Could you check a few things on this drawing? It's one solid part, dimensions in mm from its lowest x, y, z. A direction names the side the tool comes from. Give positions to 0.01 mm unless a question says otherwise; leave off trailing zeros. Write each loop counter-clockwise with the first axis right and the second up, starting at its lowest first coordinate (ties: lowest second). Pieces come first, ordered by that corner, then holes. Notation, with made-up numbers: (-16, 54) -> (2, 54) arc R34 cw to (2, 85) -> close; hole circle Ø9 at (61, -33). An arc over 180 degrees is marked (long way). Use CSV: the item, a comma, the result in double quotes. Start each with the question number.
(1) For pin 1 Ø3.5 at (y, z) = (20, 26.5) entering from +X, with a flat end and sliding along its axis, tell me the tip position at first contact or that it passes through.
(2) If we mould it in two halves opening along Y, with no side actions, what happens to the marked faces 3, 4 and 5? For each: pulls with the +Y half, pulls with the -Y half, needs draft (parallel to the pull), parting line crosses it, or undercut.
(3) Suppose I cut it at B-B on x = 26. List the corners of the cut face in (y, z) for me, plus the area to 3 significant figures.
(4) Which directions (+Z, -Z, +X, -X, +Y, -Y) give clear straight access to the entire face, cutting with the end or side of a thin tool? Please do the marked faces 1 and 2.
(5) I need wall thicknesses on L1, parallel to Z at x = 38.4, y = 20; L2, parallel to X at y = 27, z = 17.5; L3, parallel to Y at x = 39.3, z = 13. Which ranges of each line are inside material? Lowest first, please. Write a range as [from, to].
(6) Suppose I cut it at A-A on y = 20. List the corners of the cut face in (x, z) for me, plus the area to 3 significant figures.
(7) Suppose I cut it at D-D on z = 13. List the corners of the cut face in (x, y) for me.
(8) Suppose I cut it at C-C on z = 5.5. List the corners of the cut face in (x, y) for me, plus the area to 3 significant figures.
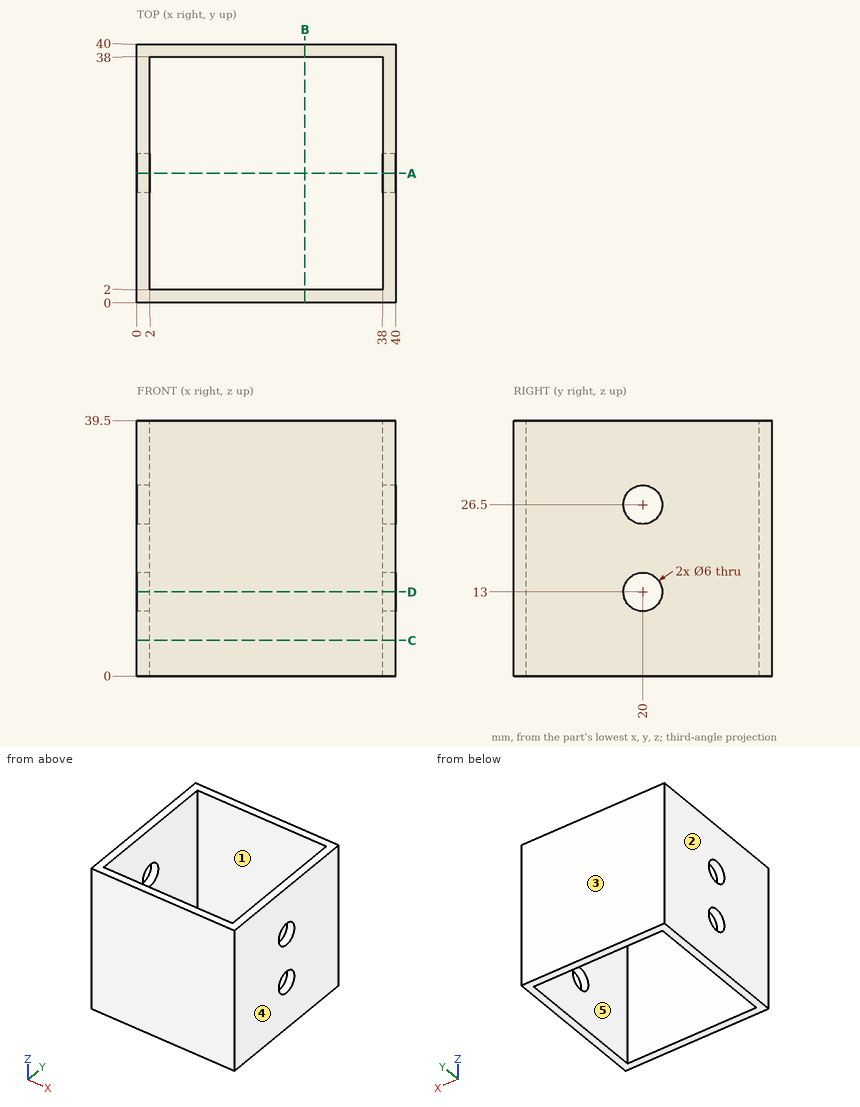
Geometry says:
1,pin 1,"through"
2,face 3,"pulls with the +Y half"
2,face 4,"needs draft"
2,face 5,"undercut"
3,outline,"(0, 0) -> (2, 0) -> (2, 39.5) -> (0, 39.5) -> close; (38, 0) -> (40, 0) -> (40, 39.5) -> (38, 39.5) -> close"
3,area,"158 mm²"
4,face 1,"+Z, -Z"
4,face 2,"+Z, -Z, -X, +Y, -Y"
5,L1,"[0, 10], [16, 23.5], [29.5, 39.5]"
5,L2,"[0, 2], [38, 40]"
5,L3,"[0, 17], [23, 40]"
6,outline,"(0, 0) -> (2, 0) -> (2, 10) -> (0, 10) -> close; (0, 16) -> (2, 16) -> (2, 23.5) -> (0, 23.5) -> close; (0, 29.5) -> (2, 29.5) -> (2, 39.5) -> (0, 39.5) -> close; (38, 0) -> (40, 0) -> (40, 10) -> (38, 10) -> close; (38, 16) -> (40, 16) -> (40, 23.5) -> (38, 23.5) -> close; (38, 29.5) -> (40, 29.5) -> (40, 39.5) -> (38, 39.5) -> close"
6,area,"110 mm²"
7,outline,"(0, 0) -> (40, 0) -> (40, 17) -> (38, 17) -> (38, 2) -> (2, 2) -> (2, 17) -> (0, 17) -> close; (0, 23) -> (2, 23) -> (2, 38) -> (38, 38) -> (38, 23) -> (40, 23) -> (40, 40) -> (0, 40) -> close"
8,outline,"(0, 0) -> (40, 0) -> (40, 40) -> (0, 40) -> close; hole (2, 2) -> (38, 2) -> (38, 38) -> (2, 38) -> close"
8,area,"304 mm²"
